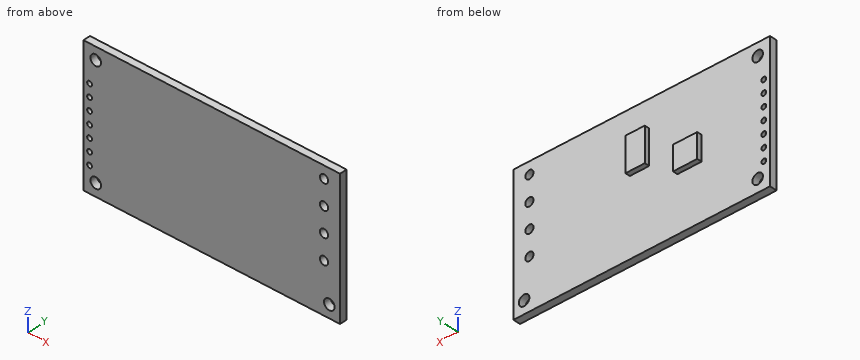
```python
from build123d import *

# Parameters (mm, degrees)
SKETCH1_W            = 53
SKETCH1_H            = 28
BOSS_EXTRUDE1_DEPTH  = 1.5
SKETCH2_R            = 1.0922
CUT_EXTRUDE1_DEPTH   = 31.008332176
LPATTERN1_COUNT      = 2
LPATTERN1_PITCH      = 22.86
LPATTERN1_COUNT_DIR2 = 2
LPATTERN1_PITCH_DIR2 = 48.26
SKETCH3_R            = 0.5
CUT_EXTRUDE2_DEPTH   = 31.008332176
LPATTERN2_COUNT      = 7
LPATTERN2_PITCH      = 2.54
SKETCH5_R            = 0.85
CUT_EXTRUDE3_DEPTH   = 31.008332176
LPATTERN4_COUNT      = 4
LPATTERN4_PITCH      = 5.08
SKETCH6_W            = 5
SKETCH6_H            = 5
SKETCH6_W_2          = 4
SKETCH6_H_2          = 7
BOSS_EXTRUDE3_DEPTH  = 1


with BuildPart() as part:
    # Sketch1 → Boss-Extrude1 (new body)
    with BuildSketch(Plane(origin=(0, 0, 0), x_dir=(1, 0, 0), z_dir=(0, 1, 0))):
        Rectangle(SKETCH1_W, SKETCH1_H)
    extrude(amount=BOSS_EXTRUDE1_DEPTH)

    # Sketch2 → Cut-Extrude1 (cut, through all)
    with BuildSketch(Plane(origin=(0, 1.5, 0), x_dir=(1, 0, 0), z_dir=(0, 1, 0))):
        with Locations(Location((-23.96, -11.46, 0), (0, 0, 270))):
            Circle(SKETCH2_R)
    cut_extrude1 = extrude(amount=-CUT_EXTRUDE1_DEPTH, mode=Mode.SUBTRACT)

    # LPattern1: Cut-Extrude1 2 × 2, 1 skipped
    with Locations(*[(j * LPATTERN1_PITCH_DIR2, 0, -i * LPATTERN1_PITCH) for i in range(LPATTERN1_COUNT) for j in range(LPATTERN1_COUNT_DIR2) if (i, j) not in ((0, 0), (0, 1))]):
        add(cut_extrude1, mode=Mode.SUBTRACT)

    # Sketch3 → Cut-Extrude2 (cut, through all)
    with BuildSketch(Plane(origin=(0, 1.5, 0), x_dir=(1, 0, 0), z_dir=(0, 1, 0))):
        with Locations(Location((-25.23, 8.739816389, 0), (0, 0, 270))):
            Circle(SKETCH3_R)
    cut_extrude2 = extrude(amount=-CUT_EXTRUDE2_DEPTH, mode=Mode.SUBTRACT)

    # LPattern2: Cut-Extrude2 ×7
    with Locations(*[(0, 0, i * LPATTERN2_PITCH) for i in range(1, LPATTERN2_COUNT)]):
        add(cut_extrude2, mode=Mode.SUBTRACT)

    # Sketch5 → Cut-Extrude3 (cut, through all)
    with BuildSketch(Plane(origin=(0, 1.5, 0), x_dir=(1, 0, 0), z_dir=(0, 1, 0))):
        with Locations(Location((23.2, -11.5, 0), (0, 0, 270))):
            Circle(SKETCH5_R)
    cut_extrude3 = extrude(amount=-CUT_EXTRUDE3_DEPTH, mode=Mode.SUBTRACT)

    # LPattern4: Cut-Extrude3 ×4
    with Locations(*[(0, 0, -i * LPATTERN4_PITCH) for i in range(1, LPATTERN4_COUNT)]):
        add(cut_extrude3, mode=Mode.SUBTRACT)

    # Sketch6 → Boss-Extrude3 (add)
    with BuildSketch(Plane(origin=(0, 1.5, 0), x_dir=(1, 0, 0), z_dir=(0, 1, 0))):
        with Locations((-9.881626536, 0.272798855)):
            Rectangle(SKETCH6_W, SKETCH6_H)
        with Locations((0.450562485, -5.004455937)):
            Rectangle(SKETCH6_W_2, SKETCH6_H_2)
    extrude(amount=BOSS_EXTRUDE3_DEPTH)


solid = part.part
```
Here's how the part is built. I have some questions about the finished solid (model axes, mm). Coordinates: 2 decimals unless noted, no trailing zeros. Order: outer loops, then holes, each group sorted by start corner. A loop starts at its lowest first (then second) coordinate and runs counter-clockwise, first axis right, second up.
Item 1: If we section it at B-B, the plane x = -23.96: List the corners of the cut face in (y, z) for me, then the cut area to 3 significant figures.
Response values:
outline: (0, -14) - (1.5, -14) - (1.5, -12.49) - (0, -12.49) - close; (0, -10.31) - (1.5, -10.31) - (1.5, 10.37) - (0, 10.37) - close; (0, 12.55) - (1.5, 12.55) - (1.5, 14) - (0, 14) - close
area: 35.4 mm2
Item 2: If we section it at C-C, the plane y = 0.4: Give the number of separate pieces and of enclosed holes in the cut face, then the cut area to 3 significant figures.
Response values:
separate pieces: 1
enclosed holes: 14
area: 1,460 mm2
Item 3: If we section it at D-D, the plane x = 18.5: List the corners of the cut face in (y, z) for me, then the cut area to 3 significant figures.
Response values:
outline: (0, -14) - (1.5, -14) - (1.5, 14) - (0, 14) - close
area: 42.0 mm2
Item 4: I'm going to push flat-ended pins straight in: pin 1 Ø0.5 at (y, z) = (2, 0.5) entering from -X; pin 2 Ø0.5 at (x, y) = (0.5, 2) entering from -Z; pin 3 Ø0.5 at (x, y) = (0, 2) entering from +Z. Where does each tip first touch, or does it pass through?
Response values:
pin 1: stops at x = -12.38
pin 2: stops at z = 1.5
pin 3: stops at z = 8.5
Item 5: I need wall thicknesses on probe 1 along X at (y, z) = (0.55, 1.34); probe 2 along X at (y, z) = (0.4, 11.46); probe 3 along Z at (x, y) = (24.3, 1). Which ranges of each line are inside material? Lowest first, please.
Response values:
probe 1: x = -26.5 to -25.72, -24.74 to 22.35, 24.05 to 26.5
probe 2: x = -26.5 to -25.05, -22.87 to 22.35, 24.05 to 26.5
probe 3: z = -14 to -12.49, -10.31 to 14
Item 6: If we section it at A-A, the plane z = -11.4: List the corners of the cut face in (x, y) for me.
Response values:
outline: (-26.5, 0) - (-25.05, 0) - (-25.05, 1.5) - (-26.5, 1.5) - close; (-22.87, 0) - (23.21, 0) - (23.21, 1.5) - (-22.87, 1.5) - close; (25.39, 0) - (26.5, 0) - (26.5, 1.5) - (25.39, 1.5) - close
